Job drawing, mm, ordinate dimensions from the low corner. One solid piece. A direction names the side the tool comes from. Round coordinates to 2 decimals unless told otherwise and drop trailing zeros. Loops run counter-clockwise (first coordinate to the right, second up) from the corner with the lowest first, then second, coordinate; pieces in that order, holes last.
1) Band-saw the part on C-C, the plane z = 3.5. Write the cut outline in (x, y), then the cut area to 3 significant figures.
2) 3-axis set-ups, long thin cutter, end or side, ignore diameter. For the marked faces 5, 6, 7 and 8: which of +Z, -Z, +X, -X, +Y, -Y reach the whole face in a straight line?
3) Band-saw the part on A-A, the plane x = 22.75. Write the cut outline in (y, z).
4) Mould opens along Z. For the marked faces 1, 2, 3 and 4 say: +Z half, -Z half, draft (parallel to the pull), parting line (faces both ways), or undercut.
5) Drop flat-ended pins along their axis: P1, Ø6, axis at x = 20.5, z = 10, coming from the +Y side; P2, Ø3.5, axis at y = 3, z = 9.5, coming from the +X side; P3, Ø7, axis at x = 2.5, y = 2, coming from the +Z side; P4, Ø7, axis at x = 4, z = 4, coming from the +Y side. Give the stop position or say it passes through.
6) Probe line 1 (X direction, y = 1.25, z = 3.5); line 2 (X direction, y = 13, z = 5.75); line 3 (Z direction, x = 17.75, y = 13). List the from-to ranges inside material, lowest first.
7) Band-saw the part on D-D, the plane x = 6.75. Write the cut outline in (y, z).
8) Band-saw the part on B-B, the plane y = 11.5. Write the cut outline in (x, z), then the cut area to 3 significant figures.
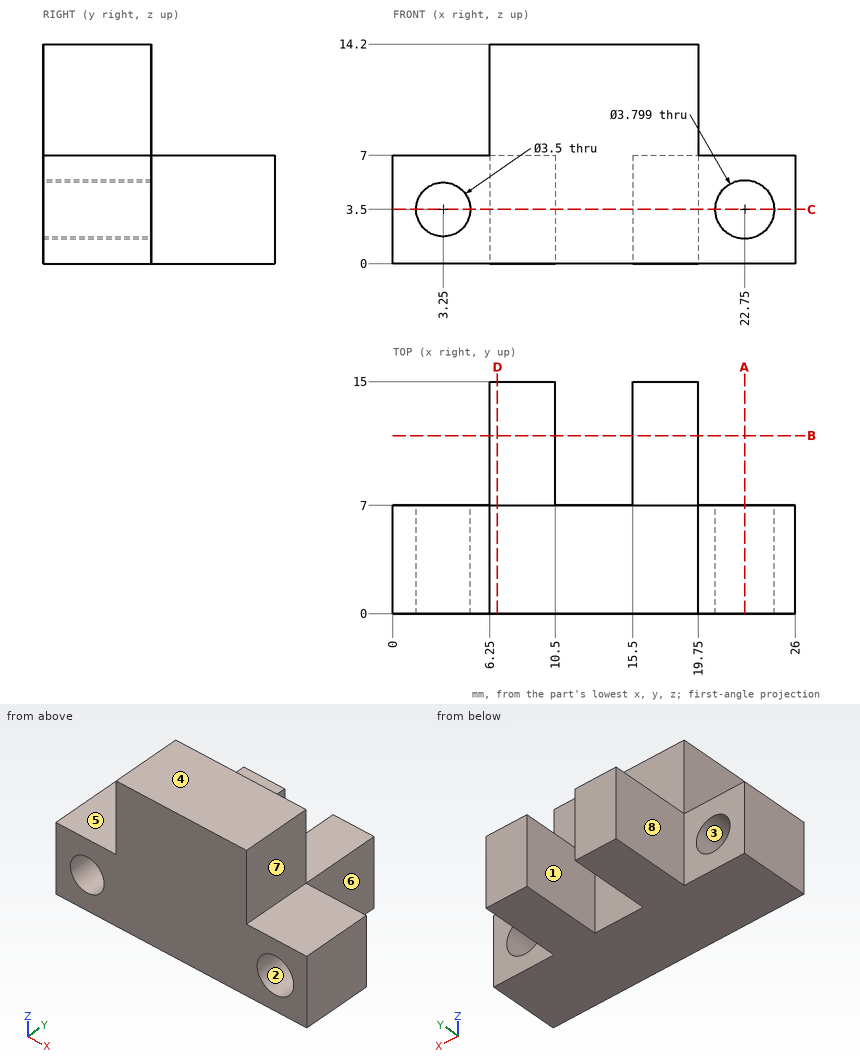
Reported:
1. outline: (0, 0) - (1.5, 0) - (1.5, 7) - (0, 7) - close; (5, 0) - (20.85, 0) - (20.85, 7) - (19.75, 7) - (19.75, 15) - (15.5, 15) - (15.5, 7) - (10.5, 7) - (10.5, 15) - (6.25, 15) - (6.25, 7) - (5, 7) - close; (24.65, 0) - (26, 0) - (26, 7) - (24.65, 7) - close
1. area: 199 mm2
2. face 5: +Z, -X, +Y, -Y
2. face 6: +Z, -Z, +X, +Y
2. face 7: +Z, +X, +Y, -Y
2. face 8: +Z, -Z, -X, +Y
3. outline: (0, 0) - (7, 0) - (7, 1.6) - (0, 1.6) - close; (0, 5.4) - (7, 5.4) - (7, 7) - (0, 7) - close
4. face 1: draft
4. face 2: undercut
4. face 3: undercut
4. face 4: +Z half
5. P1: stops at y = 7
5. P2: stops at x = 19.75
5. P3: stops at z = 7
5. P4: stops at y = 15
6. line 1: x = 0 to 1.5, 5 to 20.85, 24.65 to 26
6. line 2: x = 6.25 to 10.5, 15.5 to 19.75
6. line 3: z = 0 to 7
7. outline: (0, 0) - (15, 0) - (15, 7) - (7, 7) - (7, 14.2) - (0, 14.2) - close
8. outline: (6.25, 0) - (10.5, 0) - (10.5, 7) - (6.25, 7) - close; (15.5, 0) - (19.75, 0) - (19.75, 7) - (15.5, 7) - close
8. area: 59.5 mm2
